Design review of the part built by this model. Coordinates are the model's own, in mm. A direction names the side the tool comes from. Give positions to 0.01 mm unless a question says otherwise; leave off trailing zeros. Write each loop counter-clockwise with the first axis right and the second up, starting at its lowest first coordinate (ties: lowest second). Pieces come first, ordered by that corner, then holes. Notation, with made-up numbers: M -13,13 L 37,13 A7 ccw 37,26 Z; hole C 87,7 d7. An arc over 180 degrees is marked long. Answer in a Markdown table with one row per item.
```python
from build123d import *

# Parameters (mm, degrees)
F0_R     = 11
F1_DEPTH = 3


with BuildPart() as f1:
    # F0 (on Top) → F1 (new body)
    with BuildSketch(Plane.XY):
        with BuildLine():
            ThreePointArc((0.930703, -14.971099), (4.359901, -14.352396), (7.553815, -12.959162))
            ThreePointArc((7.553815, -12.959162), (9.025781, -11.980621), (10.37242, -10.835723))
            ThreePointArc((10.37242, -10.835723), (11.506741, -9.622625), (12.5, -8.291562))
            ThreePointArc((12.5, -8.291562), (40, 0), (12.5, 8.291562))
            ThreePointArc((12.5, 8.291562), (10.249589, 10.951983), (7.446056, 13.021377))
            ThreePointArc((7.446056, 13.021377), (5.862631, 13.806866), (4.197801, 14.400641))
            ThreePointArc((4.197801, 14.400641), (2.580067, 14.776443), (0.930703, 14.971099))
            ThreePointArc((0.930703, 14.971099), (-20, 34.641016), (-13.430703, 6.679537))
            ThreePointArc((-13.430703, 6.679537), (-14.60949, 3.400413), (-14.999871, -0.062215))
            ThreePointArc((-14.999871, -0.062215), (-14.888413, -1.826246), (-14.570222, -3.564918))
            ThreePointArc((-14.570222, -3.564918), (-14.086808, -5.153818), (-13.430703, -6.679537))
            ThreePointArc((-13.430703, -6.679537), (-20, -34.641016), (0.930703, -14.971099))
        make_face()
        with Locations((-12.5, -21.650635)):
            Circle(F0_R, mode=Mode.SUBTRACT)
        with BuildLine():
            ThreePointArc((7.606442, -7.946197), (6.618906, -8.785788), (5.539465, -9.503385))
            ThreePointArc((5.539465, -9.503385), (-4.299263, -10.125035), (-10.684829, -2.614273))
            ThreePointArc((-10.684829, -2.614273), (-10.918169, -1.339247), (-10.999905, -0.045624))
            ThreePointArc((-10.999905, -0.045624), (-6.618906, 8.785788), (3.078388, 10.56047))
            ThreePointArc((3.078388, 10.56047), (4.299263, 10.125035), (5.460441, 9.54901))
            ThreePointArc((5.460441, 9.54901), (9.514853, 5.519744), (11, 0))
            ThreePointArc((11, 0), (10.116097, -4.320251), (7.606442, -7.946197))
        make_face(mode=Mode.SUBTRACT)
        with BuildLine():
            ThreePointArc((36, 0), (25, -11), (14, 0))
            ThreePointArc((14, 0), (25, 11), (36, 0))
        make_face(mode=Mode.SUBTRACT)
        with Locations((-12.5, 21.650635)):
            Circle(F0_R, mode=Mode.SUBTRACT)
    extrude(amount=F1_DEPTH)


solid = f1.part
```
1) Add section B-B (x = 25). Write out the cut boundary in (y, z).
Geometry says:
| item | result |
|---|---|
| outline | M -15,0 L -11,0 L -11,3 L -15,3 Z; M 11,0 L 15,0 L 15,3 L 11,3 Z |
2) Add section C-C (y = 1.5). Write out the cut boundary in (x, z).
Geometry says:
| item | result |
|---|---|
| outline | M -14.92,0 L -10.9,0 L -10.9,3 L -14.92,3 Z; M 10.9,0 L 14.1,0 L 14.1,3 L 10.9,3 Z; M 35.9,0 L 39.92,0 L 39.92,3 L 35.9,3 Z |
3) The part is to be moulded in two halves that separate along X. For faces 4 (the face through (10.285, 10.919, 1.479)), 5 (the face through (-14.89, -1.8, 1.48)), 6 (the face through (-4, 11, 0)), say which applies: released by +X, released by -X, zero draft, split by the parting line, or undercut.
Geometry says:
| item | result |
|---|---|
| face 4 | undercut |
| face 5 | released by -X |
| face 6 | zero draft |
4) For faces 1 (the face through (-4, 11, 3)), 2 (the face through (-4.17, -10.18, 1.48)), 3 (the face through (5.885, 13.797, 1.479)), list the 3-axis set-ups (+Z, -Z, +X, -X, +Y, -Y) from which the entire face can be reached by the end or side of a thin tool; tool diameter is ignored.
Geometry says:
| item | result |
|---|---|
| face 1 | +Z, +X, -X, +Y, -Y |
| face 2 | +Z, -Z |
| face 3 | +Z, -Z, +Y |
5) Add section A-A (x = -12.5). Write out the cut boundary in (y, z).
Geometry says:
| item | result |
|---|---|
| outline | M -36.65,0 L -32.65,0 L -32.65,3 L -36.65,3 Z; M -10.65,0 L 10.65,0 L 10.65,3 L -10.65,3 Z; M 32.65,0 L 36.65,0 L 36.65,3 L 32.65,3 Z |
6) Insertion check: P1, Ø1, axis at y = -27, z = 2, coming from the -X side; P2, Ø1.5, axis at x = -19, z = 0.5, coming from the -Y side; P3, Ø20, axis at x = -12.5, y = -21.65, coming from the +Z side; P4, Ø1, axis at x = 1, z = 1.5, coming from the +Y side. Each pin has a flat end and moves straight along its axis. Give the tip position at first contact, or say it passes through.
Geometry says:
| item | result |
|---|---|
| P1 | x = -26.69 |
| P2 | y = -35.5 |
| P3 | through |
| P4 | y = 29.13 |
7) Add section D-D (z = 0.75). Write out the cut boundary in (x, y), and give its area (3 significant figures).
Geometry says:
| item | result |
|---|---|
| outline | M -15,-0.06 A15 ccw -14.57,-3.56 A15 ccw -13.43,-6.68 A15 ccw long 0.93,-14.97 A15 ccw 7.55,-12.96 A15 ccw 10.37,-10.84 A15 ccw 12.5,-8.29 A15 ccw long 12.5,8.29 A15 ccw 7.45,13.02 A15 ccw 4.2,14.4 A15 ccw 0.93,14.97 A15 ccw long -13.43,6.68 A15 ccw Z; hole C -12.5,-21.65 d22; hole C -12.5,21.65 d22; hole M -11,-0.05 A11 ccw -10.68,-2.61 A11 ccw 5.54,-9.5 A11 ccw 7.61,-7.95 A11 ccw 11,0 A11 ccw 5.46,9.55 A11 ccw 3.08,10.56 A11 ccw Z; hole C 25,0 d22 |
| area | 1,140 mm^2 |
8) To check wall thickness, follow probe 1 along Y at (x, z) = (25.5, 2.35); probe 2 along Y at (x, z) = (-12.5, 1.4); probe 3 along X at (y, z) = (-13.5, 1.45). State the ranges of each line that lie inside material, in increasing order. Write a range as [from, to].
Geometry says:
| item | result |
|---|---|
| probe 1 | [-14.99, -10.99], [10.99, 14.99] |
| probe 2 | [-36.65, -32.65], [-10.65, 10.65], [32.65, 36.65] |
| probe 3 | [-25.09, -19.89], [-5.11, 6.54], [18.46, 31.54] |
